Geometry check sheet. Reference: drawing and pictorial views, mm from the part's lowest x, y, z. A direction names the side the tool comes from. Round coordinates to 2 decimals unless told otherwise and drop trailing zeros. Write each loop counter-clockwise with the first axis right and the second up, starting at its lowest first coordinate (ties: lowest second). Pieces come first, ordered by that corner, then holes. Notation, with made-up numbers: (-13.5, -21) - (14.5, -21) arc R14 ccw to (14.5, -17) - close; hole circle Ø8 at (60.25, 41.25). An arc over 180 degrees is marked (long way). Use one line per item in the form item = value. Start each with the question number.
1) Section check B-B (z = 13.5). Record the boundary of the cut face in (x, y).
2) Scan lines: probe 1 along X at (y, z) = (3.75, 1) (1 decimal); probe 2 along Z at (x, y) = (15, 6.25); probe 3 along X at (y, z) = (2, 1.5). Record each from-to range of solid material in increasing order.
3) Draft check along Y on the marked faces 1 and 2. Enter one of: +Y half, -Y half, draft (parallel to the pull), parting line (faces both ways), or undercut.
4) Set-up check for the marked faces 3 and 4: record each of +Z, -Z, +X, -X, +Y, -Y from which the full face is reachable in a straight line by a thin tool's end or side.
5) Section check C-C (y = 6.25). Record the boundary of the cut face in (x, z).
6) Section check D-D (x = 17.25). Record the boundary of the cut face in (y, z).
7) Gauge pin test, flat ends, axial feed: P1, Ø1, axis at x = 8.5, z = 16.5, coming from the +Y side; P2, Ø1, axis at y = 9, z = 4, coming from the -X side; P3, Ø2, axis at x = 10.5, z = 20.5, coming from the +Y side. Record the tip position at first contact, or that the pin passes through.
8) Section check A-A (x = 10). Record the boundary of the cut face in (y, z), then the cut area to 3 significant figures.
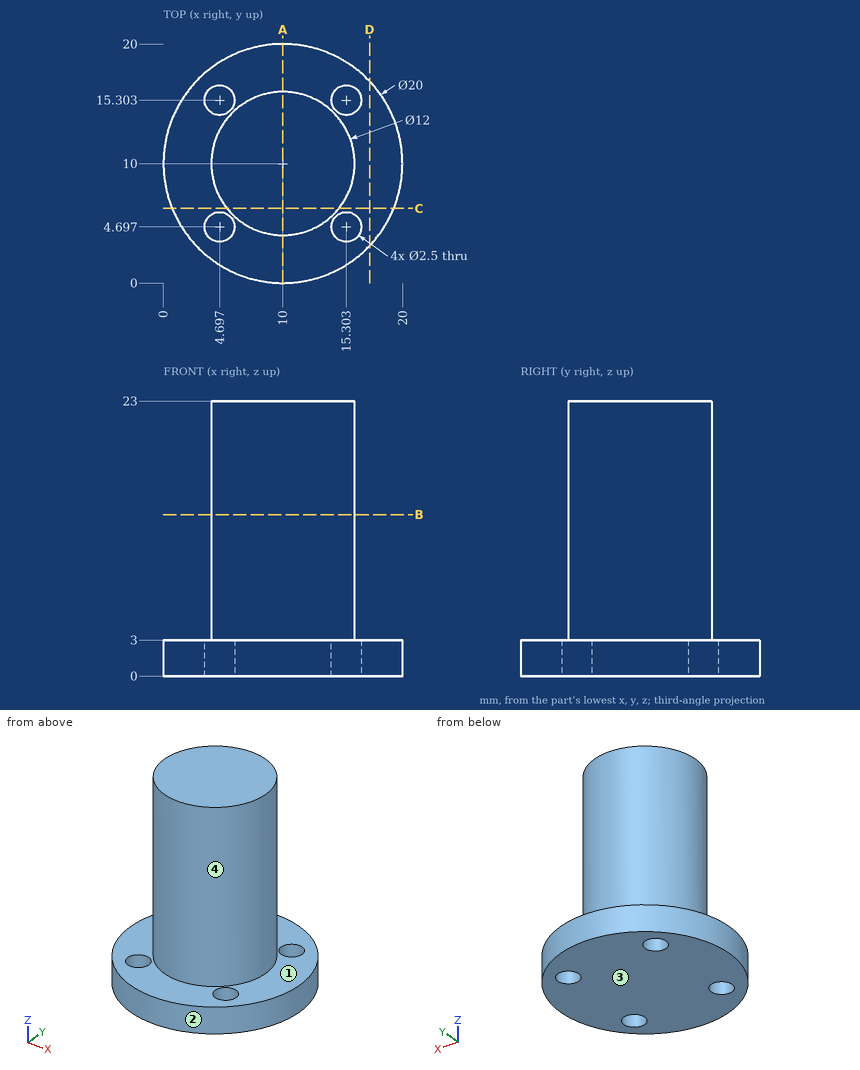
Results are:
q1.outline = circle Ø12 at (10, 10)
q2.probe_1 = 2.2 to 3.9, 5.5 to 14.5, 16.1 to 17.8
q2.probe_2 = 0 to 3
q2.probe_3 = 4 to 16
q3.face_1 = draft
q3.face_2 = parting line
q4.face_3 = -Z, +X, -X, +Y, -Y
q4.face_4 = +Z
q5.outline = (0.73, 0) - (19.27, 0) - (19.27, 3) - (14.68, 3) - (14.68, 23) - (5.32, 23) - (5.32, 3) - (0.73, 3) - close
q6.outline = (3.11, 0) - (16.89, 0) - (16.89, 3) - (3.11, 3) - close
q7.P1 = 15.92
q7.P2 = 4.02
q7.P3 = 16
q8.outline = (0, 0) - (20, 0) - (20, 3) - (16, 3) - (16, 23) - (4, 23) - (4, 3) - (0, 3) - close
q8.area = 300 mm²
